Check sheet for the modelled part. Datum: model origin and axes. Units: mm. Face numbers are marked on the shaded views. A direction names the side the tool comes from. Give positions to 0.01 mm unless a question says otherwise; leave off trailing zeros. Loops run counter-clockwise (first coordinate to the right, second up) from the corner with the lowest first, then second, coordinate; pieces in that order, holes last. Notation, with made-up numbers: M 49,-9.75 L 71,-9.75 A33 cw 71,27.25 Z; hole C 16,4 d7. An arc over 180 degrees is marked long. Use one line per item in the form item = value.
from build123d import *

# Parameters (mm, degrees)
SKETCH1_R           = 30.5
BOSS_EXTRUDE1_DEPTH = 5
SKETCH2_R           = 15.75
CUT_EXTRUDE1_DEPTH  = 2.5
SKETCH3_R           = 15.75
BOSS_EXTRUDE2_DEPTH = 2.5
SKETCH4_R           = 3.25
CUT_EXTRUDE2_DEPTH  = 5.08
SKETCH5_R           = 3.25
CUT_EXTRUDE3_DEPTH  = 5.08
SKETCH6_R           = 3.25
CUT_EXTRUDE4_DEPTH  = 5.08
BOSS_EXTRUDE3_DEPTH = 5.08
SKETCH8_W           = 25.4
SKETCH8_H           = 7.62
BOSS_EXTRUDE4_DEPTH = 25.4
SKETCH9_W           = 25.4
SKETCH9_H           = 3.81
BOSS_EXTRUDE5_DEPTH = 20.32
CUT_EXTRUDE5_DEPTH  = 7.62
SKETCH11_R          = 4.826
CUT_EXTRUDE6_DEPTH  = 2.54


with BuildPart() as part:
    # Sketch1 → Boss-Extrude1 (new body)
    with BuildSketch(Plane(origin=(0, 0, 0), x_dir=(1, 0, 0), z_dir=(0, 1, 0))):
        with Locations(Location((0, 0, 0), (0, 0, 270))):
            Circle(SKETCH1_R)
    extrude(amount=BOSS_EXTRUDE1_DEPTH)

    # Sketch2 → Cut-Extrude1 (cut)
    with BuildSketch(Plane(origin=(0, 5, 0), x_dir=(1, 0, 0), z_dir=(0, 1, 0))):
        with Locations(Location((0, 0, 0), (0, 0, 270))):
            Circle(SKETCH2_R)
    extrude(amount=-CUT_EXTRUDE1_DEPTH, mode=Mode.SUBTRACT)

    # Sketch3 → Boss-Extrude2 (add)
    with BuildSketch(Plane.XZ):
        with Locations(Location((0, 0, 0), (0, 0, 90))):
            Circle(SKETCH3_R)
    extrude(amount=BOSS_EXTRUDE2_DEPTH)

    # Sketch4 → Cut-Extrude2 (cut)
    with BuildSketch(Plane(origin=(0, 0, 0), x_dir=(-1, 0, 0), z_dir=(0, -1, 0))):
        with Locations(Location((0, 25, 0), (0, 0, 90))):
            Circle(SKETCH4_R)
    extrude(amount=-CUT_EXTRUDE2_DEPTH, mode=Mode.SUBTRACT)

    # Sketch5 → Cut-Extrude3 (cut)
    with BuildSketch(Plane.XZ):
        with Locations(Location((0, 25, 0), (0, 0, 270))):
            Circle(SKETCH5_R)
    extrude(amount=-CUT_EXTRUDE3_DEPTH, mode=Mode.SUBTRACT)

    # Sketch6 → Cut-Extrude4 (cut)
    with BuildSketch(Plane.XZ):
        with Locations(Location((17.674476483, 17.680862, 0), (0, 0, 270))):
            Circle(SKETCH6_R)
    extrude(amount=-CUT_EXTRUDE4_DEPTH, mode=Mode.SUBTRACT)

    # Sketch7 → Boss-Extrude3 (add)
    with BuildSketch(Plane(origin=(0, 0, 0), x_dir=(-1, 0, 0), z_dir=(0, -1, 0))):
        with BuildLine():
            ThreePointArc((12.7, -27.73012802), (6.499272859, -29.79948745), (0, -30.5))
            ThreePointArc((0, -30.5), (-6.499272859, -29.79948745), (-12.7, -27.73012802))
            Line((-12.7, -27.73012802), (-12.7, -65.83012802))
            Line((-12.7, -65.83012802), (12.7, -65.83012802))
            Line((12.7, -65.83012802), (12.7, -27.73012802))
        make_face()
    extrude(amount=-BOSS_EXTRUDE3_DEPTH)

    # Sketch8 → Boss-Extrude4 (add)
    with BuildSketch(Plane.XZ):
        with Locations((0, 62.02012802)):
            Rectangle(SKETCH8_W, SKETCH8_H)
    extrude(amount=BOSS_EXTRUDE4_DEPTH)

    # Sketch9 → Boss-Extrude5 (add)
    with BuildSketch(Plane.XY.offset(65.83012802)):
        with Locations((0, -23.495)):
            Rectangle(SKETCH9_W, SKETCH9_H)
    extrude(amount=BOSS_EXTRUDE5_DEPTH)

    # Sketch10 → Cut-Extrude5 (cut)
    with BuildSketch(Plane(origin=(0, 0, 58.21012802), x_dir=(-1, 0, 0), z_dir=(0, 0, -1))):
        with BuildLine():
            ThreePointArc((0, -8.128), (-3.302, -11.43), (0, -14.732))
            Line((0, -14.732), (0, -8.128))
        make_face()
        with BuildLine():
            Line((0, -8.128), (0, -14.732))
            ThreePointArc((0, -14.732), (2.334866591, -13.764866591), (3.302, -11.43))
            ThreePointArc((3.302, -11.43), (2.334866591, -9.095133409), (0, -8.128))
        make_face()
    extrude(amount=-CUT_EXTRUDE5_DEPTH, mode=Mode.SUBTRACT)

    # Sketch11 → Cut-Extrude6 (cut)
    with BuildSketch(Plane(origin=(0, 0, 58.21012802), x_dir=(-1, 0, 0), z_dir=(0, 0, -1))):
        with Locations((0, -11.43)):
            Circle(SKETCH11_R)
    extrude(amount=-CUT_EXTRUDE6_DEPTH, mode=Mode.SUBTRACT)


solid = part.part
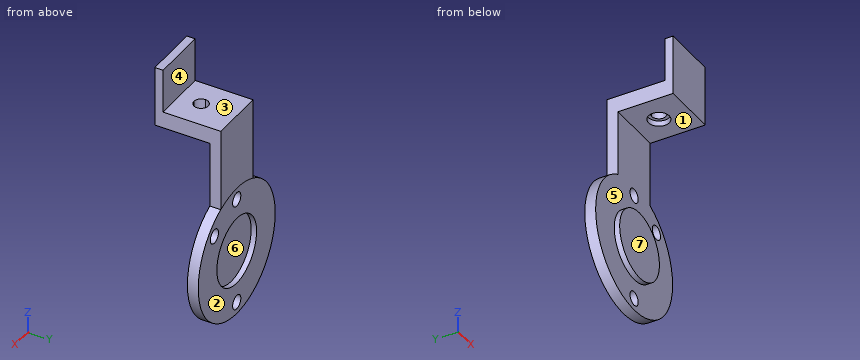
1) Section check C-C (x = -11). Record the cut outline in (y, z), then the cut area to 3 significant figures.
Evaluation:
outline = M -25.4,58.21 L 0,58.21 L 0,11.27 L -2.5,11.27 L -2.5,-11.27 L 0,-11.27 L 0,-28.45 L 5,-28.45 L 5,-11.27 L 2.5,-11.27 L 2.5,11.27 L 5,11.27 L 5,28.45 L 5.08,28.45 L 5.08,65.83 L -21.59,65.83 L -21.59,86.15 L -25.4,86.15 Z
area = 745 mm^2
2) Section check D-D (y = -4). Record the cut outline in (x, z).
Evaluation:
outline = M -12.7,58.21 L 12.7,58.21 L 12.7,65.83 L -12.7,65.83 Z
3) Set-up check for the marked faces 4, 5, 6 and 7: record each of +Z, -Z, +X, -X, +Y, -Y from which the full face is reachable in a straight line by a thin tool's end or side.
Evaluation:
face_4 = +Z, +X, -X, +Y
face_5 = -Y
face_6 = +Y
face_7 = -Z, +X, -X, -Y
4) Release check for a two-part mould opening along Z. For the marked faces 1, 2 and 3 record: pulls with the +Z half, pulls with the -Z half, needs draft (parallel to the pull), parting line crosses it, or undercut.
Evaluation:
face_1 = undercut
face_2 = needs draft
face_3 = pulls with the +Z half
5) Scan lines: line 1 (X direction, y = 3, z = 0); line 2 (Y direction, x = 1.5, z = 17.5); line 3 (Z direction, x = 7, y = -8). Record each from-to range of solid material in increasing order.
Evaluation:
line_1 = -30.5 to -15.75, 15.75 to 30.5
line_2 = 0 to 5
line_3 = 58.21 to 65.83
6) Section check B-B (z = 0). Record the cut outline in (x, y), then the cut area to 3 significant figures.
Evaluation:
outline = M -30.5,0 L -15.75,0 L -15.75,-2.5 L 15.75,-2.5 L 15.75,0 L 30.5,0 L 30.5,5 L 15.75,5 L 15.75,2.5 L -15.75,2.5 L -15.75,5 L -30.5,5 Z
area = 305 mm^2
7) Depth check by flat-ended pin: pin 1 Ø6 at (x, y) = (10.5, -10.5) entering from -Z; pin 2 Ø3 at (y, z) = (-12, 60) entering from +X; pin 3 Ø10 at (x, y) = (-20, -18) entering from +Z; pin 4 Ø25 at (x, z) = (3.5, 2) entering from -Y. Enter the tip coordinate at first touch or a pass-through.
Evaluation:
pin_1 = 58.21
pin_2 = 12.7
pin_3 = through
pin_4 = -2.5
8) Section check A-A (z = -25). Record the cut outline in (x, y), then the cut area to 3 significant figures.
Evaluation:
outline = M -17.47,0 L -3.25,0 L -3.25,5 L -17.47,5 Z; M 3.25,0 L 17.47,0 L 17.47,5 L 3.25,5 Z
area = 142 mm^2
